```python
from build123d import *

# Parameters (mm, degrees)
F1_DEPTH      = 20
F1_DEPTH_BACK = 20
F2_DEPTH      = 14
F2_DEPTH_BACK = 14
F4_DEPTH      = 25
F5_ANGLE      = 90
F6_R          = 1


with BuildPart() as f1:
    # F0 (on Right) → F1 (new body, two sides)
    with BuildSketch(Plane.YZ) as f1_sk:
        Polygon((48.225797835, 46), (-67.774202165, 46), (-67.774202165, 0), (62.225797835, 0), (62.225797835, 46), align=None)
        Polygon((62.225797835, 0), (-67.774202165, 0), (-67.774202165, -46), (48.225797835, -46), (62.225797835, -46), align=None)
    extrude(amount=F1_DEPTH)
    extrude(f1_sk.sketch, amount=-F1_DEPTH_BACK)

    # F0 (on Right) → F2 (join, two sides)
    with BuildSketch(Plane.YZ) as f2_sk:
        Polygon((55.225797835, 60), (48.225797835, 46), (62.225797835, 46), (62.225797835, 60), align=None)
        Polygon((62.225797835, -60), (62.225797835, -46), (48.225797835, -46), (55.225797835, -60), align=None)
    extrude(amount=F2_DEPTH)
    extrude(f2_sk.sketch, amount=-F2_DEPTH_BACK)

    # F3 (on face) → F4 (cut)
    with BuildSketch(Plane(origin=(0, 62.225797835, 0), x_dir=(-1, 0, 0), z_dir=(0, 1, 0))):
        with BuildLine():
            Line((2.5, 55), (2.5, 60))
            Line((2.5, 60), (-2.5, 60))
            Line((-2.5, 60), (-2.5, 55))
            ThreePointArc((-2.5, 55), (0, 52.5), (2.5, 55))
        make_face()
        with BuildLine():
            Line((2.5, -60), (2.5, -55))
            ThreePointArc((2.5, -55), (0, -52.5), (-2.5, -55))
            Line((-2.5, -55), (-2.5, -60))
            Line((-2.5, -60), (2.5, -60))
        make_face()
    extrude(amount=-F4_DEPTH, mode=Mode.SUBTRACT)


with BuildPart() as f1_1:
    # F5: moved
    add(f1.part.rotate(Axis((0, -67.774202165, 46), (-1, 0, 0)), F5_ANGLE))

    # F6
    f6_edges = [f1_1.edges().sort_by_distance(p)[0] for p in [
        (0, -159.774202, 46),
        (0, -67.774202, 46),
        (-20, -113.774202, 46),
        (20, -113.774202, 46),
    ]]
    fillet(f6_edges, radius=F6_R)


solid = f1_1.part
```
Geometry check sheet. Reference: the model listing, model coordinates, mm. A direction names the side the tool comes from. Coordinates: 2 decimals unless noted, no trailing zeros. Loops run counter-clockwise (first coordinate to the right, second up) from the corner with the lowest first, then second, coordinate; pieces in that order, holes last.
Item 1: Sectioned sample at C-C, the plane y = -161.5. Record the boundary of the cut face in (x, z).
Item 2: Sectioned sample at A-A, the plane x = 4. Record the boundary of the cut face in (y, z), then the cut area to 3 significant figures.
Item 3: Release check for a two-part mould opening along X. For faces 1 (the face through (-14, -61, -78)), 2 (the face through (0.055, -61.274, -78.7)), 3 (the face through (-8, -173.774, -80)) record: released by +X, released by -X, zero draft, split by the parting line, or undercut.
Item 4: Access from +Z, -Z, +X, -X, +Y, -Y to the whole of each face (thin tool, end or side, straight path). Record for faces 4 (the face through (14, -61, -78)), 5 (the face through (-20, -113, -19)), 6 (the face through (-14, -167, -78)), 7 (the face through (-2.5, -171, -80)), 8 (the face through (2.5, -56, -80)).
Item 5: Go/stop test with flat-tipped pins: pin 1 Ø1 at (x, z) = (-10.5, 15) entering from -Y; pin 2 Ø4 at (y, z) = (-168.5, -79.5) entering from -X; pin 3 Ø1.5 at (y, z) = (-171.5, -80.5) entering from +X. Record where each tip stops, or that it passes through.
Item 6: Sectioned sample at B-B, the plane z = -61.5. Record the boundary of the cut face in (x, y).
Item 7: Thickness scan on line 1 (Y direction, x = 11, z = 37); line 2 (Z direction, x = 13, y = -165). Record the ranges inside material, lowest first.
Check result:
1. outline: (-14, -84) - (14, -84) - (14, -70.86) - (-14, -70.86) - close
2. outline: (-173.77, -84) - (-53.77, -84) - (-53.77, -77) - (-67.77, -70) - (-67.77, 45) arc R1 ccw to (-68.77, 46) - (-158.77, 46) arc R1 ccw to (-159.77, 45) - (-159.77, -70) - (-173.77, -77) - close
2. area: 12,300 mm2
3. face 1: released by -X
3. face 2: undercut
3. face 3: zero draft
4. face 4: +Z, -Z, +X, +Y
4. face 5: +Z, -Z, -X, +Y, -Y
4. face 6: +Z, -Z, -X, -Y
4. face 7: +Z, -Z, -Y
4. face 8: +Z, -Z, +Y
5. pin 1: stops at y = -159.77
5. pin 2: stops at x = -14
5. pin 3: stops at x = 14
6. outline: (-20, -159.77) - (20, -159.77) - (20, -67.77) - (-20, -67.77) - close
7. line 1: y = -159.77 to -67.77
7. line 2: z = -84 to -72.61
